Model file for the job. Use its own axes, mm. A direction names the side the tool comes from. Round coordinates to 2 decimals unless told otherwise and drop trailing zeros. Order: outer loops, then holes, each group sorted by start corner. A loop starts at its lowest first (then second) coordinate and runs counter-clockwise, first axis right, second up. Notation, with made-up numbers: (-32, 35.5) - (8, 35.5) arc R27 ccw to (8, 60.5) - close; hole circle Ø10 at (56, 77). An arc over 180 degrees is marked (long way). Write item = value, one per line.
```python
from build123d import *

# Parameters (mm, degrees)
F0_W     = 120
F0_H     = 100
F1_DEPTH = 100
F2_T     = -4
F3_W     = 338.13595726
F3_H     = 20
F3_W_2   = 120
F3_W_3   = 358.1296569666
F4_DEPTH = 5


with BuildPart() as f1:
    # F0 (on Top) → F1 (new body)
    with BuildSketch(Plane.XY):
        with Locations((-34.0641250794, 31.4384140074)):
            Rectangle(F0_W, F0_H)
    extrude(amount=F1_DEPTH)

    # F2
    f2_openings = [f1.faces().sort_by_distance(p)[0] for p in [
        (-34.064125, 31.438414, 100),
    ]]
    offset(amount=F2_T, openings=f2_openings)

    # F3 (on face) → F4 (join)
    with BuildSketch(Plane(origin=(0, 81.4384140074, 0), x_dir=(-1, 0, 0), z_dir=(0, 1, 0))):
        with Locations((263.1321037094, 60)):
            Rectangle(F3_W, F3_H)
        with Locations((34.0641250794, 60)):
            Rectangle(F3_W_2, F3_H)
        with Locations((-205.0007034039, 60)):
            Rectangle(F3_W_3, F3_H)
    extrude(amount=-F4_DEPTH)


solid = f1.part
```
1) Cut at C-C (y = 53.5). Write the cut outline in (x, z), and give its area (3 significant figures).
Conclusion:
outline = (-94.06, 0) - (25.94, 0) - (25.94, 100) - (21.94, 100) - (21.94, 4) - (-90.06, 4) - (-90.06, 100) - (-94.06, 100) - close
area = 1,250 mm^2
2) Mould opens along Y. For faces 5 (the face through (21.936, 31, 51)), 6 (the face through (-35, -18.562, 49)), 7 (the face through (25.936, 31, 49)) say: +Y half, -Y half, draft (parallel to the pull), parting line (faces both ways), or undercut.
Conclusion:
face_5 = undercut
face_6 = -Y half
face_7 = draft
3) Wall check: line 1 along X through (y, z) = (35, 36.5); line 2 along Y through (x, z) = (-66, 31.5); line 3 along Y through (x, z) = (-76, 63.5). Give the ranges that are in metal, low to high.
Conclusion:
line_1 = -94.06 to -90.06, 21.94 to 25.94
line_2 = -18.56 to -14.56, 77.44 to 81.44
line_3 = -18.56 to -14.56, 76.44 to 81.44
4) Cut at D-D (x = -212). Write the cut outline in (y, z).
Conclusion:
outline = (76.44, 50) - (81.44, 50) - (81.44, 70) - (76.44, 70) - close
5) Cut at A-A (z = 81.5). Write the cut outline in (x, y), and give its area (3 significant figures).
Conclusion:
outline = (-94.06, -18.56) - (25.94, -18.56) - (25.94, 81.44) - (-94.06, 81.44) - close; hole (-90.06, -14.56) - (21.94, -14.56) - (21.94, 77.44) - (-90.06, 77.44) - close
area = 1,700 mm^2
6) Cut at B-B (x = -45). Write the cut outline in (y, z), and give its area (3 significant figures).
Conclusion:
outline = (-18.56, 0) - (81.44, 0) - (81.44, 100) - (77.44, 100) - (77.44, 70) - (76.44, 70) - (76.44, 50) - (77.44, 50) - (77.44, 4) - (-14.56, 4) - (-14.56, 100) - (-18.56, 100) - close
area = 1,190 mm^2
7) Flat gauge pins, fed straight in: pin 1 Ø10 at (x, z) = (-293, 55.5) entering from -Y; pin 2 Ø12 at (y, z) = (16, 39) entering from -X; pin 3 Ø4 at (x, y) = (134, 79) entering from +Z. Where does each tip first touch, or does it go through?
Conclusion:
pin_1 = 76.44
pin_2 = -94.06
pin_3 = 70
8) 3-axis set-ups, long thin cutter, end or side, ignore diameter. For faces 1 (the face through (-35, 77.438, 27)), 2 (the face through (208, 76.438, 60)), 3 (the face through (-261, 76.438, 60)), 4 (the face through (-35, -14.562, 51)): which of +Z, -Z, +X, -X, +Y, -Y reach the whole face in a straight line?
Conclusion:
face_1 = none
face_2 = +Z, -Z, +X, -Y
face_3 = +Z, -Z, -X, -Y
face_4 = +Z
